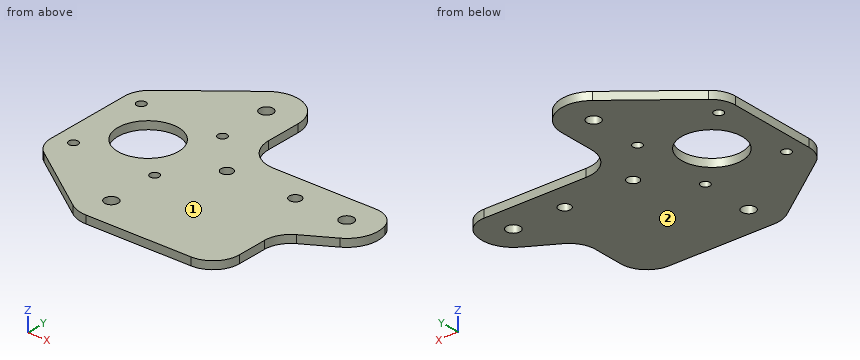
```python
from build123d import *

# Parameters (mm, degrees)
SKETCH1_R           = 2.6
SKETCH1_R_2         = 2.25
SKETCH1_R_3         = 11.5
SKETCH1_R_4         = 2.55
SKETCH1_R_5         = 2.250902383
SKETCH1_R_6         = 1.75
BOSS_EXTRUDE1_DEPTH = 3


with BuildPart() as part:
    # Sketch1 → Boss-Extrude1 (new body)
    with BuildSketch(Plane.XY):
        with BuildLine():
            Line((-17.667944903, 51.26061463), (-17.667944903, 17.69061463))
            ThreePointArc((-17.667944903, 17.69061463), (-16.55108605, 13.098251038), (-13.449984231, 9.531691833))
            Line((-13.449984231, 9.531691833), (13.449984231, -9.531691833))
            ThreePointArc((13.449984231, -9.531691833), (16.610185866, -11.106844514), (20.099329458, -11.648930616))
            Line((20.099329458, -11.648930616), (60.099329458, -11.648930616))
            ThreePointArc((60.099329458, -11.648930616), (67.17039727, -8.719998428), (70.099329458, -1.648930616))
            Line((70.099329458, -1.648930616), (70.099329458, 9.901069384))
            ThreePointArc((70.099329458, 9.901069384), (71.430361969, 14.885946781), (75.069129992, 18.543817403))
            Line((75.069129992, 18.543817403), (86.131847457, 24.98247272))
            ThreePointArc((86.131847457, 24.98247272), (91.358121472, 31.21181519), (91.413130529, 39.342966504))
            ThreePointArc((91.413130529, 39.342966504), (88.124648594, 43.697057203), (82.924988705, 45.351069384))
            Line((82.924988705, 45.351069384), (44.094988705, 45.351069384))
            ThreePointArc((44.094988705, 45.351069384), (35.609707331, 48.86578801), (32.094988705, 57.351069384))
            Line((32.094988705, 57.351069384), (32.094988705, 70.851069384))
            ThreePointArc((32.094988705, 70.851069384), (25.300553143, 81.663196782), (12.611305558, 80.231607031))
            Line((12.611305558, 80.231607031), (-13.904347525, 59.077729336))
            ThreePointArc((-13.904347525, 59.077729336), (-16.678051068, 55.598584995), (-17.667944903, 51.26061463))
        make_face()
        with Locations((80.59476396, 34.780670506)):
            Circle(SKETCH1_R, mode=Mode.SUBTRACT)
        with Locations((60.58476396, 35.351069384)):
            Circle(SKETCH1_R_2, mode=Mode.SUBTRACT)
        with Locations((4.592055097, 35.34829978)):
            Circle(SKETCH1_R_3, mode=Mode.SUBTRACT)
        with Locations((19.994988754, 70.850970592)):
            Circle(SKETCH1_R_4, mode=Mode.SUBTRACT)
        with Locations((34.584765763, 35.341387282)):
            Circle(SKETCH1_R_5, mode=Mode.SUBTRACT)
        with Locations((20.199329409, -0.149029408)):
            Circle(SKETCH1_R_4, mode=Mode.SUBTRACT)
        with Locations((19.992055097, 19.851069384)):
            Circle(SKETCH1_R_6, mode=Mode.SUBTRACT)
        with Locations((-10.907944903, 19.851069384)):
            Circle(SKETCH1_R_6, mode=Mode.SUBTRACT)
        with Locations((-10.907944903, 50.851069384)):
            Circle(SKETCH1_R_6, mode=Mode.SUBTRACT)
        with Locations((19.992055097, 50.851069384)):
            Circle(SKETCH1_R_6, mode=Mode.SUBTRACT)
    extrude(amount=BOSS_EXTRUDE1_DEPTH)


solid = part.part
```
The listing builds one solid part. Answer for the finished solid, in the listing's coordinates (mm). Face numbers are marked on the shaded views. Give positions to 0.01 mm unless a question says otherwise; leave off trailing zeros. Loops run counter-clockwise (first coordinate to the right, second up) from the corner with the lowest first, then second, coordinate; pieces in that order, holes last. Notation, with made-up numbers: (21, 36.5) - (68, 36.5) arc R19 ccw to (68, 66.5) - close; hole circle Ø2 at (67, -37.5). An arc over 180 degrees is marked (long way). Answer as CSV lines item,"result". Start each with the question number.
Item 1: A cutting plane is placed at B-B on x = 7.5. Determine the outline of the cut face in (y, z).
Item 2: A cutting plane is placed at A-A on y = 43. Determine the outline of the cut face in (x, z).
Item 3: Find the intervals of material crossed by line 1 (X direction, y = 19.5, z = 1); line 2 (X direction, y = 50, z = 2.25); line 3 (Y direction, x = 50, z = 1), in increasing order. Write a range as from..to.
Item 4: Each of these flat-tipped pins is pushed along its axis until it touches: pin 1 (0.9 mm diameter, centred on y = 3, z = 2, fed in from +X); pin 2 (1.5 mm diameter, centred on y = 39, z = 0.5, fed in from +X); pin 3 (0.9 mm diameter, centred on x = 60.5, z = 1, fed in from +Y). Where does it stop, or does it pass through?
Item 5: The mould has two halves that part along Z. Classify the marked faces 1 and 2: +Z half, -Z half, draft (parallel to the pull), parting line (faces both ways), or undercut.
Item 6: A cutting plane is placed at C-C on z = 1.95. Count the separate pieces of the cut face and the enclosed holes in it, then the cut area to 3 significant figures.
Item 7: A cutting plane is placed at D-D on y = 77.5. Determine the outline of the cut face in (x, z).
Found:
1,outline,"(-5.32, 0) - (24.22, 0) - (24.22, 3) - (-5.32, 3) - close; (46.47, 0) - (76.15, 0) - (76.15, 3) - (46.47, 3) - close"
2,outline,"(-17.67, 0) - (-3.99, 0) - (-3.99, 3) - (-17.67, 3) - close; (13.18, 0) - (88.99, 0) - (88.99, 3) - (13.18, 3) - close"
3,line 1,"x = -17.67..-12.62, -9.19..18.28, 21.71..76.71"
3,line 2,"x = -17.67..-12.44, -9.38..18.46, 21.52..34.61"
3,line 3,"y = -11.65..45.35"
4,pin 1,"stops at x = 70.1"
4,pin 2,"stops at x = 91.74"
4,pin 3,"stops at y = 45.35"
5,face 1,"+Z half"
5,face 2,"-Z half"
6,separate pieces,"1"
6,enclosed holes,"10"
6,area,"5,920 mm^2"
7,outline,"(9.19, 0) - (30.08, 0) - (30.08, 3) - (9.19, 3) - close"
